Here's how the part is built. I have some questions about the finished solid (model axes, mm). Face numbers are marked on the shaded views. Give positions to 0.01 mm unless a question says otherwise; leave off trailing zeros. Write each loop counter-clockwise with the first axis right and the second up, starting at its lowest first coordinate (ties: lowest second). Pieces come first, ordered by that corner, then holes. Notation, with made-up numbers: (82.25, 27.5) - (118.25, 27.5) arc R22 ccw to (118.25, 61.5) - close; hole circle Ø7 at (11.25, 6.5). An arc over 180 degrees is marked (long way). Use a Markdown table: item, result.
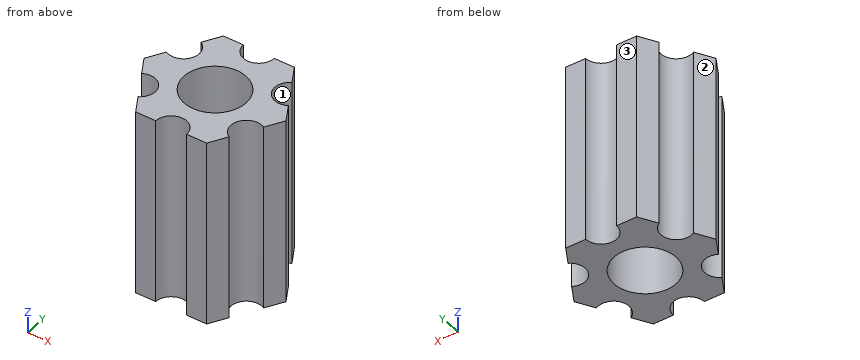
```python
from build123d import *

# Parameters (mm, degrees)
SKETCH1_R           = 2.9337
BOSS_EXTRUDE1_DEPTH = 19.325
MOVE_FACE1_BY       = 0.254


with BuildPart() as part:
    # Sketch1 → Boss-Extrude1 (new body)
    with BuildSketch(Plane(origin=(0, 0, 0), x_dir=(-1, 0, 0), z_dir=(0, 0, -1))):
        with BuildLine():
            Line((-4.703606334, -4.55311485), (-3.666174209, -6.35))
            Line((-3.666174209, -6.35), (-1.591309959, -6.35))
            ThreePointArc((-1.591309959, -6.35), (0, -4.758690041), (1.591309959, -6.35))
            Line((1.591309959, -6.35), (3.666174209, -6.35))
            Line((3.666174209, -6.35), (4.703606334, -4.55311485))
            ThreePointArc((4.703606334, -4.55311485), (4.121146464, -2.37934502), (6.294916294, -1.79688515))
            Line((6.294916294, -1.79688515), (7.332348419, 0))
            Line((7.332348419, 0), (6.294916294, 1.79688515))
            ThreePointArc((6.294916294, 1.79688515), (4.121146464, 2.37934502), (4.703606334, 4.55311485))
            Line((4.703606334, 4.55311485), (3.666174209, 6.35))
            Line((3.666174209, 6.35), (1.591309959, 6.35))
            ThreePointArc((1.591309959, 6.35), (0, 4.758690041), (-1.591309959, 6.35))
            Line((-1.591309959, 6.35), (-3.666174209, 6.35))
            Line((-3.666174209, 6.35), (-4.703606334, 4.55311485))
            ThreePointArc((-4.703606334, 4.55311485), (-4.121146464, 2.37934502), (-6.294916294, 1.79688515))
            Line((-6.294916294, 1.79688515), (-7.332348419, 0))
            Line((-7.332348419, 0), (-6.294916294, -1.79688515))
            ThreePointArc((-6.294916294, -1.79688515), (-4.121146464, -2.37934502), (-4.703606334, -4.55311485))
        make_face()
        with Locations(Location((0, 0, 0), (0, 0, 180))):
            Circle(SKETCH1_R, mode=Mode.SUBTRACT)
    extrude(amount=-BOSS_EXTRUDE1_DEPTH)

    # Move Face1: a curved face moved inward by 0.254
    add(Solid.thicken(part.faces().sort_by_distance((-2.9337, 0, 9.6625))[0], -MOVE_FACE1_BY), mode=Mode.SUBTRACT)


solid = part.part
```
Item 1: Will these pins go through, and if not, where does the flat tip stop? pin 1 Ø3 at (y, z) = (2, 15) entering from +X; pin 2 Ø1 at (x, z) = (-6, 9) entering from -Y.
Values:
| item | result |
|---|---|
| pin 1 | stops at x = 7.04 |
| pin 2 | stops at y = -1.8 |
Item 2: I need wall thicknesses on line 1 along Y through (x, z) = (0, 9.5); line 2 along Y through (x, z) = (-2.75, 1.5); line 3 along Y through (x, z) = (-4.5, 17.25). Which ranges of each line are inside material? Lowest first, please. Write a range as [from, to].
Values:
| item | result |
|---|---|
| line 1 | y = [-4.76, -3.19], [3.19, 4.76] |
| line 2 | y = [-6.35, -1.61], [1.61, 6.35] |
| line 3 | y = [-4.91, -4.41], [-1.94, 1.94], [4.41, 4.91] |
Item 3: If we section it at C-C, the plane y = 2.5: Write out the boundary of the cut face in (x, z) (3 decimals).
Values:
| item | result |
|---|---|
| outline | (-4.058, 0) - (-1.978, 0) - (-1.978, 19.325) - (-4.058, 19.325) - close; (1.978, 0) - (4.058, 0) - (4.058, 19.325) - (1.978, 19.325) - close |
Item 4: Thinking about a two-plate mould opening in X: for the marked faces 1, 2 and 3, which applies, +X half, -X half, draft (parallel to the pull), parting line (faces both ways), or undercut?
Values:
| item | result |
|---|---|
| face 1 | undercut |
| face 2 | -X half |
| face 3 | draft |
Item 5: If we section it at A-A, the plane x = 0: Write out the boundary of the cut face in (y, z) (3 decimals), plus the area to 3 significant figures.
Values:
| item | result |
|---|---|
| outline | (-4.759, 0) - (-3.188, 0) - (-3.188, 19.325) - (-4.759, 19.325) - close; (3.188, 0) - (4.759, 0) - (4.759, 19.325) - (3.188, 19.325) - close |
| area | 60.7 mm2 |
Item 6: If we section it at B-B, the plane z = 3: Write out the boundary of the cut face in (x, y) (3 decimals), plus the area to 3 significant figures.
Values:
| item | result |
|---|---|
| outline | (-7.332, 0) - (-6.295, -1.797) arc R1.591 cw to (-4.704, -4.553) - (-3.666, -6.35) - (-1.591, -6.35) arc R1.591 cw to (1.591, -6.35) - (3.666, -6.35) - (4.704, -4.553) arc R1.591 cw to (6.295, -1.797) - (7.332, 0) - (6.295, 1.797) arc R1.591 cw to (4.704, 4.553) - (3.666, 6.35) - (1.591, 6.35) arc R1.591 cw to (-1.591, 6.35) - (-3.666, 6.35) - (-4.704, 4.553) arc R1.591 cw to (-6.295, 1.797) - close; hole circle Ø6.375 at (0, 0) |
| area | 83.9 mm2 |
Item 7: If we section it at D-D, the plane x = -4.25: Write out the boundary of the cut face in (y, z) (3 decimals), plus the area to 3 significant figures.
Values:
| item | result |
|---|---|
| outline | (-5.339, 0) - (-4.161, 0) - (-4.161, 19.325) - (-5.339, 19.325) - close; (-2.189, 0) - (2.189, 0) - (2.189, 19.325) - (-2.189, 19.325) - close; (4.161, 0) - (5.339, 0) - (5.339, 19.325) - (4.161, 19.325) - close |
| area | 130 mm2 |
